Design review of the part shown in the three views and the two pictorial views. Dimensions are in mm from the part's minimum x, y and z. A direction names the side the tool comes from. Coordinates: 2 decimals unless noted, no trailing zeros. Order: outer loops, then holes, each group sorted by start corner. A loop starts at its lowest first (then second) coordinate and runs counter-clockwise, first axis right, second up. Notation, with made-up numbers: (67, 21.25) -> (120, 21.25) arc R7 ccw to (120, 31.25) -> close; hole circle Ø9 at (42, 45.25). An arc over 180 degrees is marked (long way). Answer as CSV lines item,"result". Start each with the question number.
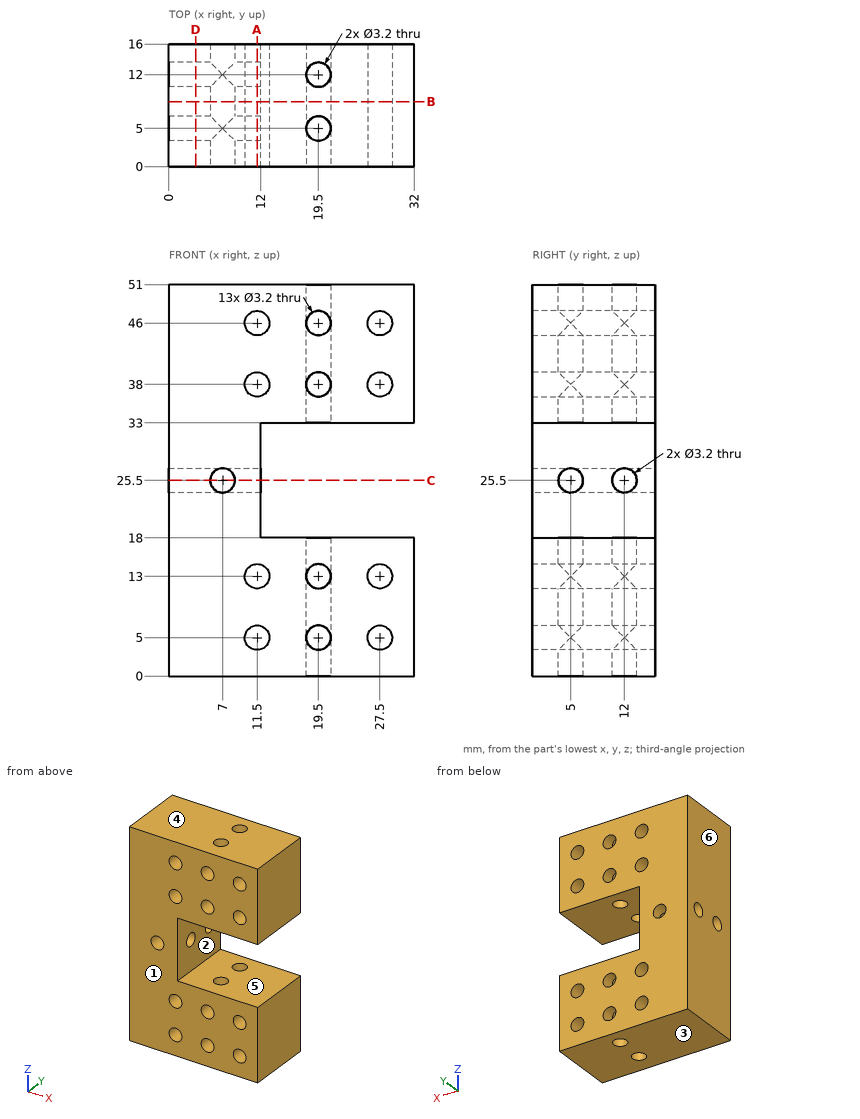
1) Consider section C-C (z = 25.5). Give the boundary of the cut face in (x, y).
2) Insertion check: pin 1 Ø2 at (y, z) = (4, 28) entering from +X. The pin has a flat end and moves straight along its axis. Give the tip position at first contact, or say it passes through.
3) Consider section D-D (x = 3.5). Give the boundary of the cut face in (y, z).
4) Tool access review of the marked faces 1 and 2: name each direction out of +Z, -Z, +X, -X, +Y, -Y from which nothing blocks a thin tool from reaching the whole face with its end or side.
5) Mouldability with a two-part tool opening along Z and no side actions: class the marked faces 3, 4, 5 and 6 as released by +Z, released by -Z, zero draft, split by the parting line, or undercut.
6) Wall thickness on L1, parallel to X at y = 11, z = 46; L2, parallel to X at y = 12, z = 1.8; L3, parallel to Y at x = 19, z = 36: over which ranges is each line inside the solid? List them lowest first. Write a range as [from, to].
7) Consider section A-A (x = 11.5). Give the boundary of the cut face in (y, z).
8) Consider section B-B (y = 8.5). Count the separate pieces of the cut face and the enclosed holes in it, plus the area to 3 significant figures.
Result:
1,outline,"(0, 0) -> (5.4, 0) -> (5.4, 3.4) -> (0, 3.4) -> close; (0, 6.6) -> (5.4, 6.6) -> (5.4, 10.4) -> (0, 10.4) -> close; (0, 13.6) -> (5.4, 13.6) -> (5.4, 16) -> (0, 16) -> close; (8.6, 0) -> (12, 0) -> (12, 3.4) -> (8.6, 3.4) -> close; (8.6, 6.6) -> (12, 6.6) -> (12, 10.4) -> (8.6, 10.4) -> close; (8.6, 13.6) -> (12, 13.6) -> (12, 16) -> (8.6, 16) -> close"
2,pin 1,"x = 12"
3,outline,"(0, 0) -> (16, 0) -> (16, 51) -> (0, 51) -> close; hole circle Ø3.2 at (5, 25.5); hole circle Ø3.2 at (12, 25.5)"
4,face 1,"+Z, -Z, +X, -X, -Y"
4,face 2,"+X, +Y, -Y"
5,face 3,"released by -Z"
5,face 4,"released by +Z"
5,face 5,"undercut"
5,face 6,"zero draft"
6,L1,"[0, 9.9], [13.1, 17.9], [21.1, 25.9], [29.1, 32]"
6,L2,"[0, 17.9], [21.1, 32]"
6,L3,"[0, 3.48], [6.52, 10.48], [13.52, 16]"
7,outline,"(0, 0) -> (16, 0) -> (16, 3.4) -> (0, 3.4) -> close; (0, 6.6) -> (16, 6.6) -> (16, 11.4) -> (0, 11.4) -> close; (0, 14.6) -> (16, 14.6) -> (16, 36.4) -> (0, 36.4) -> close; (0, 39.6) -> (16, 39.6) -> (16, 44.4) -> (0, 44.4) -> close; (0, 47.6) -> (16, 47.6) -> (16, 51) -> (0, 51) -> close; hole circle Ø3.2 at (5, 25.5); hole circle Ø3.2 at (12, 25.5)"
8,separate pieces,"1"
8,enclosed holes,"13"
8,area,"1,230 mm2"
